The model under review builds one solid part; all positions refer to its coordinate system, in mm. Coordinates: 2 decimals unless noted, no trailing zeros. Loops run counter-clockwise (first coordinate to the right, second up) from the corner with the lowest first, then second, coordinate; pieces in that order, holes last. Notation, with made-up numbers: M 79,0.25 L 101,0.25 A30 cw 101,34.25 Z; hole C -14.75,-24 d2. An arc over 180 degrees is marked long. Write item = value, one per line. Start each with the question number.
Q1. Clearance check with flat-ended pins moving along their axes: pin 1 Ø3 at (x, y) = (-5, -24) entering from -Z; pin 2 Ø1 at (x, y) = (6.5, 26) entering from -Z; pin 3 Ø1.5 at (x, y) = (2, -35) entering from +Z. State where each tip first meets the part, or that it passes through.
Q2. We need section A-A on y = 96.5. Give the boundary of the cut face in (x, z).
Q3. We need section B-B on z = 3.75. Give the boundary of the cut face in (x, y).
Q4. Wall thickness on probe 1 along X at (y, z) = (-134.5, -1); probe 2 along Z at (x, y) = (-0.25, -100.5); probe 3 along X at (y, z) = (46, 3.75): over which ranges is each line inside the solid? List them lowest first.
from build123d import *

# Parameters (mm, degrees)
SKETCH1_R           = 10
BOSS_EXTRUDE1_DEPTH = 160
CUT_EXTRUDE1_DEPTH  = 40


with BuildPart() as part:
    # Sketch1 → Boss-Extrude1 (new, symmetric)
    with BuildSketch(Plane(origin=(0, 0, 0), x_dir=(1, 0, 0), z_dir=(0, 1, 0))):
        with Locations(Location((0, 0, 0), (0, 0, 270))):
            Circle(SKETCH1_R)
    extrude(amount=BOSS_EXTRUDE1_DEPTH, both=True)

    # Sketch2 → Cut-Extrude1 (cut)
    with BuildSketch(Plane(origin=(0, 160, 0), x_dir=(1, 0, 0), z_dir=(0, 1, 0))):
        Polygon((-1.75, 9.845684334), (-1.75, 8), (1.75, 8), (1.75, 9.845684334), (1.75, 11.147310955), (-1.75, 11.147310955), align=None)
    extrude(amount=-CUT_EXTRUDE1_DEPTH, mode=Mode.SUBTRACT)


solid = part.part
Returned:
q1.pin_1 = -9.37
q1.pin_2 = -8
q1.pin_3 = 9.92
q2.outline = C 0,0 d20
q3.outline = M -9.27,-160 L 9.27,-160 L 9.27,160 L -9.27,160 Z
q4.probe_1 = -9.95 to 9.95
q4.probe_2 = -10 to 10
q4.probe_3 = -9.27 to 9.27
